Design review of the part shown in the three views and the two pictorial views. Dimensions are in mm from the part's minimum x, y and z. A direction names the side the tool comes from. Round coordinates to 2 decimals unless told otherwise and drop trailing zeros. Loops run counter-clockwise (first coordinate to the right, second up) from the corner with the lowest first, then second, coordinate; pieces in that order, holes last. Notation, with made-up numbers: M 53.25,-33 L 99.25,-33 A26 cw 99.25,-17 Z; hole C 17,88.25 d9. An arc over 180 degrees is marked long. Answer as CSV lines item,"result". Start each with the question number.
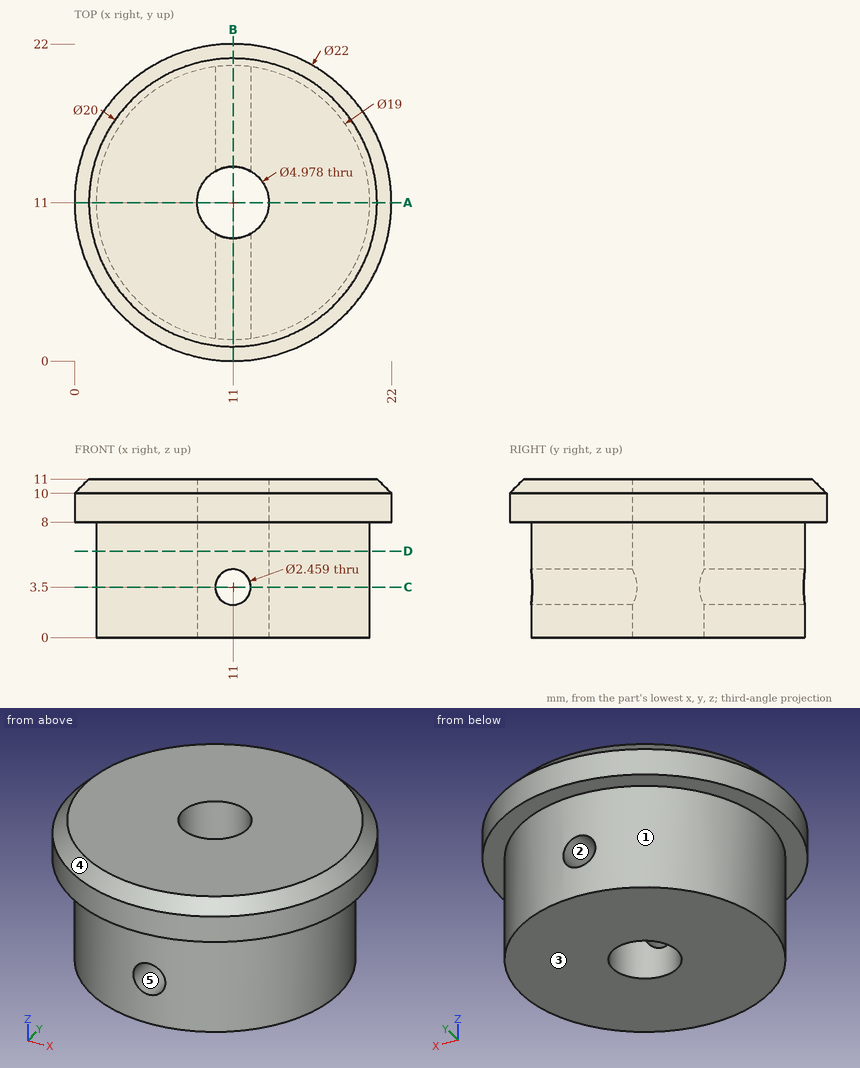
Item 1: Insertion check: pin 1 Ø2 at (y, z) = (6, 3) entering from +X; pin 2 Ø5 at (x, z) = (10.5, 3) entering from +Y; pin 3 Ø2 at (y, z) = (7.5, 4) entering from -X; pin 4 Ø4.5 at (x, y) = (11, 11) entering from +Z. Each pin has a flat end and moves straight along its axis. Give the tip position at first contact, or say it passes through.
Item 2: Consider section A-A, the plane y = 11. Write out the cut boundary in (x, z).
Item 3: Consider section D-D, the plane z = 6. Write out the cut boundary in (x, y), then the cut area to 3 significant figures.
Item 4: Consider section C-C, the plane z = 3.5. Write out the cut boundary in (x, y).
Item 5: The part is to be moulded in two halves that separate along Z. For the marked faces 3, 4 and 5, say which applies: +Z half, -Z half, draft (parallel to the pull), parting line (faces both ways), or undercut.
Item 6: Consider section B-B, the plane x = 11. Write out the cut boundary in (y, z), then the cut area to 3 significant figures.
Item 7: To check wall thickness, follow line 1 (Z direction, x = 11, y = 17); line 2 (Y direction, x = 11, z = 6.25); line 3 (Z direction, x = 10.5, y = 6.25). State the ranges of each line that lie inside material, in increasing order.
Item 8: Tool access review of the marked faces 1 and 2: name each direction out of +Z, -Z, +X, -X, +Y, -Y from which nothing blocks a thin tool from reaching the whole face with its end or side.
Found:
1,pin 1,"stops at x = 19.62"
1,pin 2,"stops at y = 20.5"
1,pin 3,"stops at x = 1.83"
1,pin 4,"passes through"
2,outline,"M 0,8 L 1.5,8 L 1.5,0 L 8.51,0 L 8.51,11 L 1,11 L 0,10 Z; M 13.49,0 L 20.5,0 L 20.5,8 L 22,8 L 22,10 L 21,11 L 13.49,11 Z"
3,outline,"C 11,11 d19; hole C 11,11 d4.98"
3,area,"264 mm^2"
4,outline,"M 9.77,1.58 L 9.77,8.84 A2.49 cw 9.77,13.16 L 9.77,20.42 A9.5 ccw Z; M 12.23,1.58 A9.5 ccw 12.23,20.42 L 12.23,13.16 A2.49 cw 12.23,8.84 Z"
5,face 3,"-Z half"
5,face 4,"+Z half"
5,face 5,"undercut"
6,outline,"M 0,8 L 1.5,8 L 1.5,4.73 L 8.51,4.73 L 8.51,11 L 1,11 L 0,10 Z; M 1.5,0 L 8.51,0 L 8.51,2.27 L 1.5,2.27 Z; M 13.49,0 L 20.5,0 L 20.5,2.27 L 13.49,2.27 Z; M 13.49,4.73 L 20.5,4.73 L 20.5,8 L 22,8 L 22,10 L 21,11 L 13.49,11 Z"
6,area,"128 mm^2"
7,line 1,"z = 0 to 2.27, 4.73 to 11"
7,line 2,"y = 1.5 to 8.51, 13.49 to 20.5"
7,line 3,"z = 0 to 2.38, 4.62 to 11"
8,face 1,"-Z"
8,face 2,"+Y, -Y"
